Verification items for this drawing (mm, ordinates from the low corner). Give positions to 0.01 mm unless a question says otherwise; leave off trailing zeros. Order: outer loops, then holes, each group sorted by start corner. A loop starts at its lowest first (then second) coordinate and runs counter-clockwise, first axis right, second up. Notation, with made-up numbers: (37.25, 33) -> (78.25, 33) arc R12 cw to (78.25, 37) -> close; hole circle Ø11 at (10.25, 5). An arc over 180 degrees is marked (long way). One line per question, with ' | ' between items.
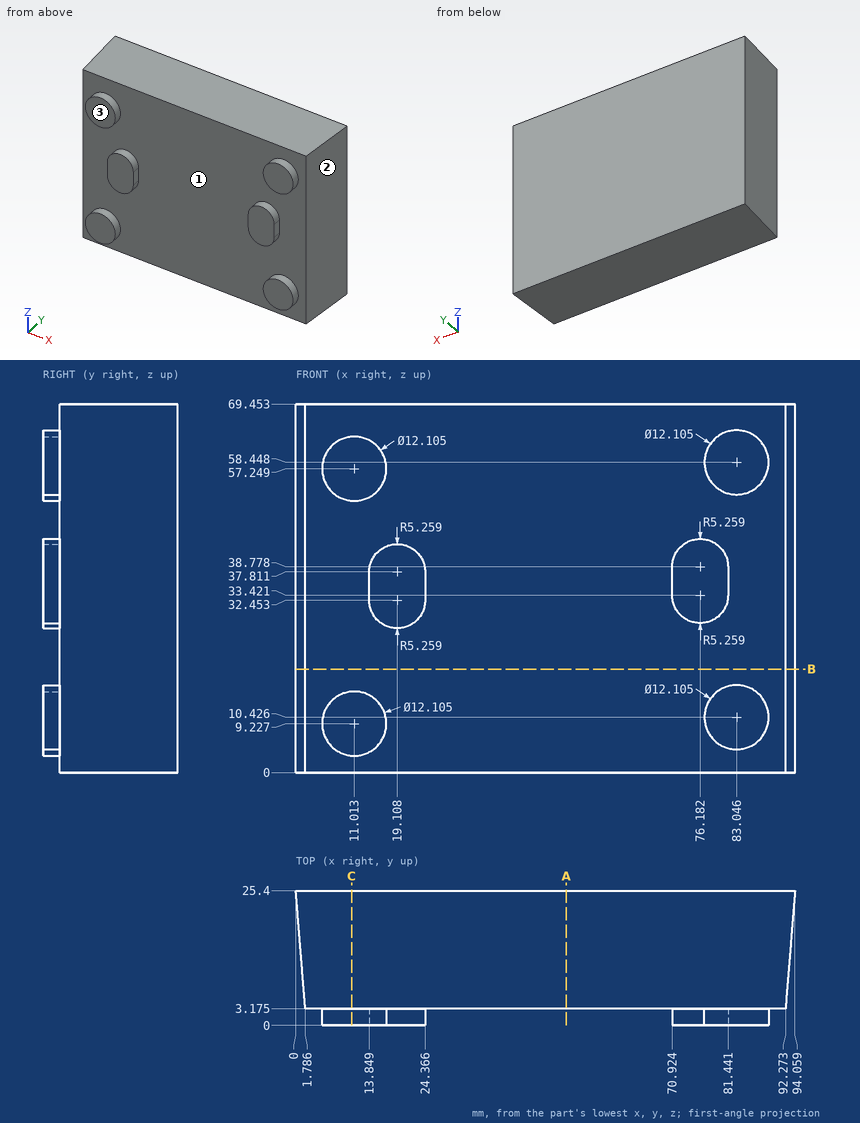
Q1. Depth check by flat-ended pin: pin 1 Ø1.5 at (y, z) = (13.5, 26.5) entering from +X; pin 2 Ø12 at (y, z) = (18.5, 16.5) entering from +X; pin 3 Ø2.5 at (y, z) = (2, 34.5) entering from -X; pin 4 Ø12 at (x, y) = (19.5, 6) entering from -Z. Enter the tip coordinate at first touch or a pass-through.
Result sheet:
pin 1: stops at x = 93.16 | pin 2: stops at x = 93.99 | pin 3: stops at x = 1.78 | pin 4: stops at z = 0
Q2. Thickness scan on line 1 (Z direction, x = 80, y = 1.25) (1 decimal); line 2 (X direction, y = 3.25, z = 63.5); line 3 (Y direction, x = 77.5, z = 25) (1 decimal). Record the ranges inside material, lowest first.
Result sheet:
line 1: z = 5.2 to 15.7, 29.8 to 42.4, 53.2 to 63.7 | line 2: x = 1.78 to 92.28 | line 3: y = 3.2 to 25.4
Q3. Mould release check, pull along X, two halves, no side actions. Record for the marked faces 1, 2 and 3: pulls with the +X half, pulls with the -X half, needs draft (parallel to the pull), parting line crosses it, or undercut.
Result sheet:
face 1: undercut | face 2: pulls with the +X half | face 3: needs draft
Q4. Section check B-B (z = 19.5). Enter the section's corners in (x, y) (1 decimal).
Result sheet:
outline: (0, 25.4) -> (1.8, 3.2) -> (92.3, 3.2) -> (94.1, 25.4) -> close
Q5. Section check A-A (x = 51). Enter the section's corners in (y, z) (1 decimal).
Result sheet:
outline: (3.2, 0) -> (25.4, 0) -> (25.4, 69.5) -> (3.2, 69.5) -> close
Q6. Section check C-C (x = 10.5). Enter the section's corners in (y, z) (1 decimal).
Result sheet:
outline: (0, 3.2) -> (3.2, 3.2) -> (3.2, 0) -> (25.4, 0) -> (25.4, 69.5) -> (3.2, 69.5) -> (3.2, 63.3) -> (0, 63.3) -> (0, 51.2) -> (3.2, 51.2) -> (3.2, 15.3) -> (0, 15.3) -> close
